The listing builds one solid part. Answer for the finished solid, in the listing's coordinates (mm). A direction names the side the tool comes from. Coordinates: 2 decimals unless noted, no trailing zeros. Loops run counter-clockwise (first coordinate to the right, second up) from the corner with the lowest first, then second, coordinate; pieces in that order, holes last. Notation, with made-up numbers: (73, 52.25) -> (107, 52.25) arc R36 cw to (107, 90.25) -> close; hole circle Ø5 at (83.5, 39.25). An arc over 180 degrees is marked (long way). Answer in a Markdown table with one row per item.
```python
from build123d import *

# Parameters (mm, degrees)
SKETCH_1_R          = 32
SKETCH_1_R_2        = 2.3
EXTRUDE_1_DEPTH     = 51
SKETCH_2_R          = 13.15
CUT_EXTRUDE_1_DEPTH = 40
CUT_EXTRUDE_START   = -10.5
SKETCH_16_R         = 36.699938781
SKETCH_16_R_2       = 25
CUT_EXTRUDE_5_DEPTH = 30
FILLET_4_R          = 8
SKETCH_17_R         = 12.5
CUT_EXTRUDE_6_DEPTH = 6
SKETCH_18_R         = 32
SKETCH_18_R_2       = 12.5
EXTRUDE_2_DEPTH     = 7.25
SKETCH_19_R         = 44
SKETCH_19_R_2       = 12.5
EXTRUDE_3_DEPTH     = 2.25
FILLET_5_R          = 8


with BuildPart() as part:
    # Эскиз1 → Бобышка-Вытянуть1 (new body)
    with BuildSketch(Plane(origin=(0, 0, 0), x_dir=(1, 0, 0), z_dir=(0, 1, 0))):
        with Locations(Location((0, 0, 0), (0, 0, 270))):
            Circle(SKETCH_1_R)
        with Locations(Location((0, 0, 0), (0, 0, 270))):
            Circle(SKETCH_1_R_2, mode=Mode.SUBTRACT)
    extrude(amount=EXTRUDE_1_DEPTH)

    # Эскиз2 → Вырез-Вытянуть1 (cut)
    with BuildSketch(Plane.XZ):
        with Locations(Location((0, 0, 0), (0, 0, 270))):
            Circle(SKETCH_2_R)
    extrude(amount=-CUT_EXTRUDE_1_DEPTH, mode=Mode.SUBTRACT)

    # Эскиз16 → Вырез-Вытянуть5 (cut)
    with BuildSketch(Plane.XZ.offset(CUT_EXTRUDE_START)):
        Circle(SKETCH_16_R)
        with Locations(Location((0, 0, 0), (0, 0, 270))):
            Circle(SKETCH_16_R_2, mode=Mode.SUBTRACT)
    extrude(amount=-CUT_EXTRUDE_5_DEPTH, mode=Mode.SUBTRACT)

    # Скругление4
    # the kernel refuses this fillet: 8 mm, written as the material it takes off along each edge
    with BuildSketch(Plane(origin=(0, 10.5, 0), x_dir=(0, 0, 1), z_dir=(1, 0, 0))) as fillet_4_piece_1:
        with BuildLine():
            CenterArc((24, 7.937253933), FILLET_4_R, 277.180755781, 82.819244219)
            Line((25, 0), (25.02, -0.158745079))
            ThreePointArc((25.02, -0.158745079), (28.5, -0.16), (32, -0.16))
            Line((32, -0.16), (32.16, 0))
            Line((32.16, 0), (32.16, 7.937253933))
            Line((32.16, 7.937253933), (32, 7.937253933))
        make_face()
    revolve(axis=Axis((0, 10.5, 0), (0, -1, 0)), mode=Mode.SUBTRACT)
    with BuildSketch(Plane(origin=(0, 40.5, 0), x_dir=(0, 0, 1), z_dir=(1, 0, 0))) as fillet_4_piece_2:
        with BuildLine():
            CenterArc((24, -7.937253933), FILLET_4_R, 0, 82.819244219)
            Line((32, -7.937253933), (32.16, -7.937253933))
            Line((32.16, -7.937253933), (32.16, 0))
            Line((32.16, 0), (32, 0.16))
            ThreePointArc((32, 0.16), (28.5, 0.16), (25.02, 0.158745079))
            Line((25.02, 0.158745079), (25, 0))
        make_face()
    revolve(axis=Axis((0, 40.5, 0), (0, -1, 0)), mode=Mode.SUBTRACT)

    # Эскиз17 → Вырез-Вытянуть6 (cut)
    with BuildSketch(Plane(origin=(0, 51, 0), x_dir=(1, 0, 0), z_dir=(0, 1, 0))):
        with Locations(Location((0, 0, 0), (0, 0, 270))):
            Circle(SKETCH_17_R)
    extrude(amount=-CUT_EXTRUDE_6_DEPTH, mode=Mode.SUBTRACT)

    # Эскиз18 → Бобышка-Вытянуть2 (add)
    with BuildSketch(Plane(origin=(0, 51, 0), x_dir=(1, 0, 0), z_dir=(0, 1, 0))):
        with Locations(Location((0, 0, 0), (0, 0, 90))):
            Circle(SKETCH_18_R)
        with Locations(Location((0, 0, 0), (0, 0, 270))):
            Circle(SKETCH_18_R_2, mode=Mode.SUBTRACT)
    extrude(amount=EXTRUDE_2_DEPTH)

    # Эскиз19 → Бобышка-Вытянуть3 (add)
    with BuildSketch(Plane(origin=(0, 58.25, 0), x_dir=(1, 0, 0), z_dir=(0, 1, 0))):
        with Locations(Location((0, 0, 0), (0, 0, 270))):
            Circle(SKETCH_19_R)
        with Locations(Location((0, 0, 0), (0, 0, 270))):
            Circle(SKETCH_19_R_2, mode=Mode.SUBTRACT)
    extrude(amount=EXTRUDE_3_DEPTH)

    # Скругление5
    fillet_5_edges = [part.edges().sort_by_distance(p)[0] for p in [
        (0, 58.25, 32),
    ]]
    fillet(fillet_5_edges, radius=FILLET_5_R)


solid = part.part
```
Item 1: Flat-ended cylindrical pins translate along their axes: pin 1 Ø1 at (x, z) = (20.5, 33.5) entering from -Y; pin 2 Ø1.5 at (x, y) = (-27, 33.5) entering from -Z; pin 3 Ø16 at (x, z) = (0, 0) entering from -Y; pin 4 Ø3 at (x, y) = (17.5, 19) entering from -Z. Find the tip coordinate at first contact, or state that the pin passes through.
Findings below:
| item | result |
|---|---|
| pin 1 | stops at y = 58.16 |
| pin 2 | passes through |
| pin 3 | stops at y = 40 |
| pin 4 | stops at z = -19.21 |
Item 2: Find the intervals of material crossed by probe 1 along X at (y, z) = (12.5, 0); probe 2 along X at (y, z) = (48.75, 0); probe 3 along Y at (x, z) = (-26, 34), in increasing order.
Findings below:
| item | result |
|---|---|
| probe 1 | x = -25 to -13.15, 13.15 to 25 |
| probe 2 | x = -32 to -12.5, 12.5 to 32 |
| probe 3 | y = 58.25 to 60.5 |
Item 3: Determine the mould class of faces 5 (the face through (-42.954, 59.359, -9.538)), 6 (the face through (-3, 45, 0)), 7 (the face through (0, 0, 14)) for opening direction Z: +Z half, -Z half, draft (parallel to the pull), parting line (faces both ways), or undercut.
Findings below:
| item | result |
|---|---|
| face 5 | parting line |
| face 6 | undercut |
| face 7 | draft |
Item 4: A cutting plane is placed at B-B, the plane y = 7. Determine the outline of the cut face in (x, z), plus the area to 3 significant figures.
Findings below:
| item | result |
|---|---|
| outline | circle Ø61.31 at (0, 0); hole circle Ø26.3 at (0, 0) |
| area | 2,410 mm2 |
Item 5: A cutting plane is placed at A-A, the plane y = 22.5. Determine the outline of the cut face in (x, z), plus the area to 3 significant figures.
Findings below:
| item | result |
|---|---|
| outline | circle Ø50 at (0, 0); hole circle Ø26.3 at (0, 0) |
| area | 1,420 mm2 |
Item 6: A tool of negligible diameter and unlimited length cuts with its end or side. For faces 1 (the face through (7.509, 25.29, -23.846)), 2 (the face through (40.1, 58.25, -3.5)), 3 (the face through (-9, 60.5, 9)), 4 (the face through (3.755, 52.642, 11.923)), from which of +Z, -Z, +X, -X, +Y, -Y can it reach the whole face along a straight path? Write none if from no direction.
Findings below:
| item | result |
|---|---|
| face 1 | none |
| face 2 | -Y |
| face 3 | +Z, -Z, +X, -X, +Y |
| face 4 | +Y |
